```python
from build123d import *

# Parameters (mm, degrees)
F0_W           = 2
F0_H           = 9
F1_DEPTH       = 25
F3_D           = 5.6134
F3_DEPTH       = 25
F3_TIP         = 1.6864354994
F5_D           = 5.6134
F5_DEPTH       = 85
F5_TIP         = 1.6864354994
F7_D           = 4.318
F7_DEPTH       = 25
F7_CSINK_D     = 7.7978
F7_CSINK_ANGLE = 82
F7_TIP         = 1.2972580765
F8_R           = 5
F9_R           = 1
F11_DEPTH      = 0.4
F12_R          = 1


# Not quite as in the source:
# - a feature names something its author has since deleted; it is built from what else it names


with BuildPart() as f1:
    # F0 (on Top) → F1 (new body)
    with BuildSketch(Plane.XY):
        Polygon((0, 166), (0, 0), (154.2796328583, 0), (154.2796328583, 9), (137.7157287525, 9), (134.8873016278, 9), (9, 9), (9, 134.8873016278), (9, 137.7157287525), (9, 138.1715728753), (9, 163.1715728753), (9, 166), align=None)
        Polygon((36.4558441227, 135.7157287525), (34.4558441227, 137.7157287525), (9, 137.7157287525), (11, 135.7157287525), align=None)
        Polygon((38.4558441227, 133.7157287525), (36.4558441227, 135.7157287525), (36.4558441227, 110.2598846298), (38.4558441227, 108.2598846298), align=None)
        Polygon((134.8873016278, 9), (137.7157287525, 9), (128.8237887356, 17.891940017), (126.8237887356, 19.891940017), (126.8236856744, 19.8920430782), (124.8236856744, 21.8920430782), (99.3678415517, 47.3478872009), (97.3678415517, 49.3478872009), (97.3677384905, 49.347990262), (95.3677384905, 51.347990262), (69.9118943678, 76.8038343848), (67.9118943678, 78.8038343848), (67.9117913066, 78.8039374459), (65.9117913066, 80.8039374459), (40.4559471839, 106.2597815687), (38.4559471839, 108.2597815687), (38.4558441227, 108.2598846298), (36.4558441227, 110.2598846298), (11, 135.7157287525), (9, 137.7157287525), (9, 134.8873016278), align=None)
        Polygon((166, 9), (9, 166), (9, 163.1715728753), (34.4558441227, 137.7157287525), (36.4558441227, 135.7157287525), (38.4558441227, 133.7157287525), (63.9117913066, 108.2597815687), (65.9117913066, 106.2597815687), (67.9117913066, 104.2597815687), (93.3677384905, 78.8038343848), (95.3677384905, 76.8038343848), (97.3677384905, 74.8038343848), (122.8236856744, 49.3478872009), (124.8236856744, 47.3478872009), (126.8236856744, 45.3478872009), (150.2702352589, 21.9013376164), (152.2796328583, 19.891940017), (154.2796328583, 17.891940017), (156.2796328583, 15.891940017), (163.1715728753, 9), align=None)
        Polygon((65.9117913066, 106.2597815687), (63.9117913066, 108.2597815687), (38.4559471839, 108.2597815687), (40.4559471839, 106.2597815687), align=None)
        Polygon((67.9117913066, 104.2597815687), (65.9117913066, 106.2597815687), (65.9117913066, 80.8039374459), (67.9117913066, 78.8039374459), align=None)
        Polygon((95.3677384905, 76.8038343848), (93.3677384905, 78.8038343848), (67.9118943678, 78.8038343848), (69.9118943678, 76.8038343848), align=None)
        Polygon((97.3677384905, 49.347990262), (97.3677384905, 74.8038343848), (95.3677384905, 76.8038343848), (95.3677384905, 51.347990262), align=None)
        Polygon((99.3678415517, 47.3478872009), (124.8236856744, 47.3478872009), (122.8236856744, 49.3478872009), (97.3678415517, 49.3478872009), align=None)
        Polygon((124.8236856744, 21.8920430782), (126.8236856744, 19.8920430782), (126.8236856744, 45.3478872009), (124.8236856744, 47.3478872009), align=None)
        Polygon((128.8237887356, 17.891940017), (154.2796328583, 17.891940017), (152.2796328583, 19.891940017), (126.8237887356, 19.891940017), align=None)
        Polygon((154.2796328583, 17.891940017), (154.2796328583, 9), (156.2796328583, 9), (156.2796328583, 15.891940017), align=None)
        with Locations((155.2796328583, 4.5)):
            Rectangle(F0_W, F0_H)
        Polygon((156.2796328583, 9), (156.2796328583, 0), (166, 0), (166, 6.1715728753), (163.1715728753, 9), align=None)
        Polygon((166, 6.1715728753), (166, 9), (163.1715728753, 9), align=None)
    extrude(amount=F1_DEPTH)

    # F3
    with Locations(Plane(origin=(0, 0, 0), x_dir=(0, -1, 0), z_dir=(-1, 0, 0))):
        with Locations((-36, 12.5)):
            Hole(F3_D / 2, depth=F3_DEPTH)
            with Locations((0, 0, -(F3_DEPTH + F3_TIP / 2))):  # 118° drill point
                Cone(0, F3_D / 2, F3_TIP, mode=Mode.SUBTRACT)

    # F5
    with Locations(Plane(origin=(0, 0, 0), x_dir=(0, -1, 0), z_dir=(-1, 0, 0))):
        with Locations((-101, 12.5)):
            Hole(F5_D / 2, depth=F5_DEPTH)
            with Locations((0, 0, -(F5_DEPTH + F5_TIP / 2))):  # 118° drill point
                Cone(0, F5_D / 2, F5_TIP, mode=Mode.SUBTRACT)

    # F7
    with Locations(Plane(origin=(0, 9, 0), x_dir=(-1, 0, 0), z_dir=(0, 1, 0))):
        with Locations((-59, 12.5)):
            CounterSinkHole(F7_D / 2, F7_CSINK_D / 2, depth=F7_DEPTH, counter_sink_angle=F7_CSINK_ANGLE)
            with Locations((0, 0, -(F7_DEPTH + F7_TIP / 2))):  # 118° drill point
                Cone(0, F7_D / 2, F7_TIP, mode=Mode.SUBTRACT)

    # F8
    f8_edges = [f1.edges().sort_by_distance(p)[0] for p in [
        (9, 9, 12.5),
    ]]
    fillet(f8_edges, radius=F8_R)

    # F9
    f9_edges = [f1.edges().sort_by_distance(p)[0] for p in [
        (166, 9, 12.5),
        (166, 0, 12.5),
        (0, 0, 12.5),
        (0, 166, 12.5),
        (9, 166, 12.5),
    ]]
    fillet(f9_edges, radius=F9_R)

    # F10 (on face) → F11 (join)
    with BuildSketch(Plane(origin=(0, 0, 0), x_dir=(1, 0, 0), z_dir=(0, 0, -1))):
        with BuildLine():
            Line((156, 5), (156, 0))
            Line((156, 0), (165, 0))
            ThreePointArc((165, 0), (165.5171897304, -0.1441292254), (165.8852951503, -0.5349704344))
            Line((165.8852951503, -0.5349704344), (166, -0.5349704344))
            Line((166, -0.5349704344), (166, 5))
            Line((166, 5), (156, 5))
        make_face()
        with BuildLine():
            Line((0, 5), (0, -1))
            ThreePointArc((0, -1), (0.2928932188, -0.2928932188), (1, 0))
            Line((1, 0), (10, 0))
            Line((10, 0), (10, 5))
            Line((10, 5), (0, 5))
        make_face()
    extrude(amount=-F11_DEPTH)

    # F12
    f12_edges = [f1.edges().sort_by_distance(p)[0] for p in [
        (166, -5, 0.2),
        (156, -5, 0.2),
        (0, -5, 0.2),
        (10, -5, 0.2),
    ]]
    fillet(f12_edges, radius=F12_R)


solid = f1.part
```
For this review, take the finished solid that the model builds, in its own axes (mm). A direction names the side the tool comes from. Round coordinates to 2 decimals unless told otherwise and drop trailing zeros. Write each loop counter-clockwise with the first axis right and the second up, starting at its lowest first coordinate (ties: lowest second). Pieces come first, ordered by that corner, then holes. Notation, with made-up numbers: (6.5, 3.5) - (39.5, 3.5) arc R9 cw to (39.5, 20.5) - close; hole circle Ø11 at (72, -14.5). An arc over 180 degrees is marked (long way). Answer as a JSON object with one key per item and string values.
1. Tool access review of faces 4 (the face through (140, 19.892, 12)), 5 (the face through (0, 82, 12)), 6 (the face through (61.06, 3.45, 13.15)): name each direction out of +Z, -Z, +X, -X, +Y, -Y from which nothing blocks a thin tool from reaching the whole face with its end or side.
Response values:
{"face 4": "+Z, -Z", "face 5": "+Z, -Z, -X, +Y, -Y", "face 6": "-Y"}
2. To check wall thickness, follow line 1 along X through (y, z) = (53, 10); line 2 along Y through (x, z) = (23, 8.5); line 3 along X through (y, z) = (125, 20.5). State the ranges of each line that lie inside material, in increasing order.
Response values:
{"line 1": "x = 0 to 9, 90.89 to 93.72, 95.37 to 97.37, 119.17 to 122", "line 2": "y = 0 to 9, 120.89 to 123.72, 135.72 to 137.72, 149.17 to 152", "line 3": "x = 0 to 9, 18.89 to 21.72, 36.46 to 38.46, 47.17 to 50"}
3. We need section A-A on y = 123. Give the boundary of the cut face in (x, z), then the cut area to 3 significant figures.
Response values:
{"outline": "(0, 0) - (9, 0) - (9, 25) - (0, 25) - close; (20.89, 0) - (23.72, 0) - (23.72, 25) - (20.89, 25) - close; (36.46, 0) - (38.46, 0) - (38.46, 25) - (36.46, 25) - close; (49.17, 0) - (52, 0) - (52, 25) - (49.17, 25) - close", "area": "416 mm2"}
4. We need section D-D on x = 20. Give the boundary of the cut face in (y, z), then the cut area to 3 significant figures.
Response values:
{"outline": "(0, 0) - (9, 0) - (9, 25) - (0, 25) - close; (123.89, 0) - (126.72, 0) - (126.72, 25) - (123.89, 25) - close; (135.72, 0) - (137.72, 0) - (137.72, 25) - (135.72, 25) - close; (152.17, 0) - (155, 0) - (155, 25) - (152.17, 25) - close", "area": "416 mm2"}
5. We need section C-C on y = 144. Give the boundary of the cut face in (x, z), then the cut area to 3 significant figures.
Response values:
{"outline": "(0, 0) - (9, 0) - (9, 25) - (0, 25) - close; (28.17, 0) - (31, 0) - (31, 25) - (28.17, 25) - close", "area": "296 mm2"}
6. We need section B-B on x = 59. Give the boundary of the cut face in (y, z).
Response values:
{"outline": "(0, 0) - (9, 0) - (9, 8.6) - (7, 10.34) - (0, 10.34) - close; (0, 14.66) - (7, 14.66) - (9, 16.4) - (9, 25) - (0, 25) - close; (84.89, 0) - (87.72, 0) - (87.72, 25) - (84.89, 25) - close; (106.26, 0) - (108.26, 0) - (108.26, 25) - (106.26, 25) - close; (113.17, 0) - (116, 0) - (116, 25) - (113.17, 25) - close"}
7. For pin 1 Ø8.5 at (x, z) = (145, 17.5) entering from +Y; pin 2 Ø12.5 at (x, z) = (27, 17) entering from +Y; pin 3 Ø12 at (x, z) = (31.5, 15) entering from -Y, all flat-tipped, find the tip position at first contact; note any pin that passes through.
Response values:
{"pin 1": "stops at y = 34.25", "pin 2": "stops at y = 154.25", "pin 3": "stops at y = 0"}
8. Draft analysis for pull direction Y (two halves, no side actions). For faces 1 (the face through (5, -3, 0.4)), 2 (the face through (75, 9, 12)), 3 (the face through (89, 86, 12)), state which applies: +Y half, -Y half, draft (parallel to the pull), parting line (faces both ways), or undercut.
Response values:
{"face 1": "draft", "face 2": "undercut", "face 3": "+Y half"}
